from build123d import *

# Parameters (mm, degrees)
SKETCH1_R           = 1.5
BOSS_EXTRUDE1_DEPTH = 5
SKETCH2_R           = 1.5
CUT_EXTRUDE1_DEPTH  = 1.75


with BuildPart() as part:
    # Sketch1 → Boss-Extrude1 (new, symmetric)
    with BuildSketch(Plane.XY):
        with BuildLine():
            Line((0, -3), (5, -3))
            ThreePointArc((5, -3), (7.121320344, -2.121320344), (8, 0))
            Line((8, 0), (8, 6))
            ThreePointArc((8, 6), (3.095785062, 12.50802611), (3.515332481, 20.646189784))
            Line((3.515332481, 20.646189784), (3, 23))
            Line((3, 23), (0, 23))
            Line((0, 23), (0, 3))
            ThreePointArc((0, 3), (-3, 0), (0, -3))
        make_face()
        Circle(SKETCH1_R, mode=Mode.SUBTRACT)
        with Locations((5, 0)):
            Circle(SKETCH1_R, mode=Mode.SUBTRACT)
    extrude(amount=BOSS_EXTRUDE1_DEPTH, both=True)

    # Sketch2 → Cut-Extrude1 (cut, symmetric)
    with BuildSketch(Plane.XY):
        with BuildLine():
            Line((0, 3.5), (5, 3.5))
            ThreePointArc((5, 3.5), (8.5, 0), (5, -3.5))
            Line((5, -3.5), (0, -3.5))
            ThreePointArc((0, -3.5), (-3.5, 0), (0, 3.5))
        make_face()
        Circle(SKETCH2_R, mode=Mode.SUBTRACT)
        with Locations((5, 0)):
            Circle(SKETCH2_R, mode=Mode.SUBTRACT)
    extrude(amount=CUT_EXTRUDE1_DEPTH, both=True, mode=Mode.SUBTRACT)


solid = part.part
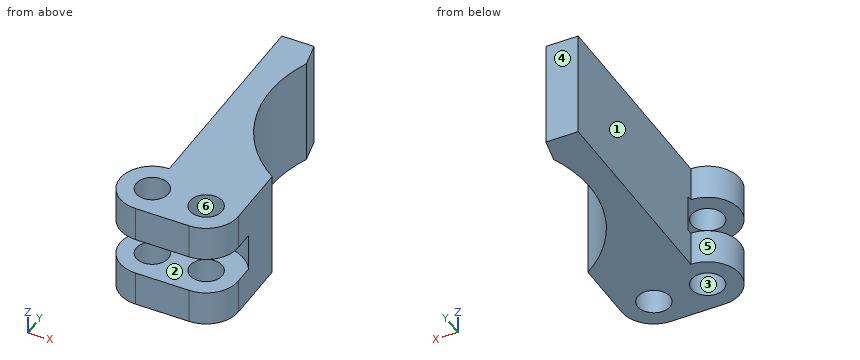
Here's how the part is built. I have some questions about the finished solid (model axes, mm). Face numbers are marked on the shaded views. A direction names the side the tool comes from. Round coordinates to 2 decimals unless told otherwise and drop trailing zeros. Write each loop counter-clockwise with the first axis right and the second up, starting at its lowest first coordinate (ties: lowest second). Pieces come first, ordered by that corner, then holes.
1. For the marked faces 1, 2 and 3, which set-ups out of +Z, -Z, +X, -X, +Y, -Y let a thin tool reach every point of the face, with its end or its side?
2. Suppose I cut it at C-C (y = 2.75). List the corners of the cut face in (x, z) for me.
3. If we mould it in two halves opening along X, with no side actions, what happens to the marked faces 4, 5 and 6? For each: released by +X, released by -X, zero draft, split by the parting line, or undercut.
4. Will these pins go through, and if not, where does the flat tip stop? pin 1 Ø4 at (x, y) = (5, 0) entering from -Z; pin 2 Ø1.8 at (x, z) = (3.5, 0.5) entering from -Y; pin 3 Ø6 at (y, z) = (9, -3) entering from -X; pin 4 Ø3 at (y, z) = (9, 3.5) entering from +X.
5. Suppose I cut it at A-A (z = 2). List the corners of the cut face in (x, y) for me, and give its area (3 significant figures).
6. Suppose I cut it at D-D (x = -1). List the corners of the cut face in (y, z) for me, and give its area (3 significant figures).
7. I need wall thicknesses on L1, parallel to Z at x = 3, y = -0.25; L2, parallel to X at y = -1, z = -2.5; L3, parallel to Y at x = 5, z = 2.6. Which ranges of each line are inside material? Lowest first, please.
8. Suppose I cut it at B-B (x = 5.5). List the corners of the cut face in (y, z) for me, and give its area (3 significant figures).
Answer sheet:
1. face 1: +Z, -Z, -X, +Y
1. face 2: -X, -Y
1. face 3: +Z, -Z
2. outline: (-1.2, -5) - (8, -5) - (8, 5) - (-1.2, 5) - (-1.2, 1.75) - (7.17, 1.75) - (7.17, -1.75) - (-1.2, -1.75) - close
3. face 4: zero draft
3. face 5: released by -X
3. face 6: undercut
4. pin 1: stops at z = -5
4. pin 2: stops at y = 3.5
4. pin 3: stops at x = 0
4. pin 4: stops at x = 6.13
5. outline: (0, -3) - (5, -3) arc R3 ccw to (8, 0) - (8, 6) arc R11.93 cw to (3.52, 20.65) - (3, 23) - (0, 23) - (0, 3) arc R3 ccw to start; hole circle Ø3 at (0, 0); hole circle Ø3 at (5, 0)
5. area: 133 mm2
6. outline: (-2.83, -5) - (-1.12, -5) - (-1.12, -1.75) - (-2.83, -1.75) - close; (-2.83, 1.75) - (-1.12, 1.75) - (-1.12, 5) - (-2.83, 5) - close; (1.12, -5) - (2.83, -5) - (2.83, -1.75) - (1.12, -1.75) - close; (1.12, 1.75) - (2.83, 1.75) - (2.83, 5) - (1.12, 5) - close
6. area: 22.2 mm2
7. L1: z = -5 to -1.75, 1.75 to 5
7. L2: x = -2.83 to -1.12, 1.12 to 3.88, 6.12 to 7.83
7. L3: y = -3 to -1.5, 1.5 to 8.79
8. outline: (-2.96, -5) - (-1.41, -5) - (-1.41, -1.75) - (-2.96, -1.75) - close; (-2.96, 1.75) - (-1.41, 1.75) - (-1.41, 5) - (-2.96, 5) - close; (1.41, -5) - (8.17, -5) - (8.17, 5) - (1.41, 5) - (1.41, 1.75) - (3.46, 1.75) - (3.46, -1.75) - (1.41, -1.75) - close
8. area: 70.5 mm2
